from build123d import *

# Parameters (mm, degrees)
SALIENTE_EXTRUIR1_DEPTH = 10
REDONDEO1_R             = 30
REDONDEO2_R             = 150
REDONDEO3_R             = 10
CORTAR_EXTRUIR1_DEPTH   = 5
CROQUIS4_R              = 2.65
CORTAR_EXTRUIR3_DEPTH   = 5


with BuildPart() as part:
    # Croquis1 → Saliente-Extruir1 (new body)
    with BuildSketch(Plane.XY):
        Polygon((0, 0), (260, 0), (274.106158457, 80), (127.13677389, 110), (50.509014114, 286.543118386), (96.75188515, 306.61463205), (64.899290737, 380), (0, 351.830749872), align=None)
    extrude(amount=SALIENTE_EXTRUIR1_DEPTH)

    # Redondeo1
    redondeo1_edges = [part.edges().sort_by_distance(p)[0] for p in [
        (50.509014114, 286.543118386, 5),
    ]]
    fillet(redondeo1_edges, radius=REDONDEO1_R)

    # Redondeo2
    redondeo2_edges = [part.edges().sort_by_distance(p)[0] for p in [
        (127.13677389, 110, 5),
    ]]
    fillet(redondeo2_edges, radius=REDONDEO2_R)

    # Redondeo3
    redondeo3_edges = [part.edges().sort_by_distance(p)[0] for p in [
        (64.899290737, 380, 5),
        (96.75188515, 306.61463205, 5),
        (274.106158457, 80, 5),
    ]]
    fillet(redondeo3_edges, radius=REDONDEO3_R)

    # Croquis2 → Cortar-Extruir1 (cut)
    with BuildSketch(Plane.XY.offset(10)):
        Polygon((39.986675692, 287.208594669), (90.439116158, 309.107253328), (88.289066035, 314.060765665), (83.517508369, 311.989692162), (59.787325531, 366.661791285), (64.558883197, 368.732864788), (62.408833074, 373.686377124), (0, 346.598099131), (0, 340.711367047), (57.402301073, 365.626581966), (81.13248391, 310.954482844), (37.836625569, 292.162107006), align=None)
    extrude(amount=-CORTAR_EXTRUIR1_DEPTH, mode=Mode.SUBTRACT)

    # Croquis4 → Cortar-Extruir3 (cut)
    with BuildSketch(Plane.XY.offset(10)):
        with Locations((132.709363959, 88.450085292)):
            Circle(CROQUIS4_R)
        with Locations((142.50732293, 86.450085292)):
            Circle(CROQUIS4_R)
        with Locations((134.109252611, 70.308111078)):
            Circle(CROQUIS4_R)
        Polygon((254.785909436, 5), (265.569150028, 66.433298656), (260.668303978, 67.433679667), (249.709468889, 5), align=None)
        with BuildLine():
            Line((240.334745072, 17.65), (246.334745072, 17.65))
            ThreePointArc((246.334745072, 17.65), (248.984745072, 15), (246.334745072, 12.35))
            Line((246.334745072, 12.35), (240.334745072, 12.35))
            ThreePointArc((240.334745072, 12.35), (237.684745072, 15), (240.334745072, 17.65))
        make_face()
        with BuildLine():
            Line((249.552515929, 67.294739764), (255.431207696, 66.094330202))
            ThreePointArc((255.431207696, 66.094330202), (257.497449003, 62.967727115), (254.370845916, 60.901485808))
            Line((254.370845916, 60.901485808), (248.49215415, 62.10189537))
            ThreePointArc((248.49215415, 62.10189537), (246.425912843, 65.228498457), (249.552515929, 67.294739764))
        make_face()
        with BuildLine():
            Line((15, 17.65), (21, 17.65))
            ThreePointArc((21, 17.65), (23.65, 15), (21, 12.35))
            Line((21, 12.35), (15, 12.35))
            ThreePointArc((15, 12.35), (12.35, 15), (15, 17.65))
        make_face()
        Polygon((99.011814836, 96.436284415), (19.818301977, 278.890655481), (24.771814314, 281.040705604), (103.965327172, 98.586334538), align=None)
        with BuildLine():
            Line((13.6, 178.915374936), (13.6, 172.915374936))
            ThreePointArc((13.6, 172.915374936), (16.25, 170.265374936), (18.9, 172.915374936))
            Line((18.9, 172.915374936), (18.9, 178.915374936))
            ThreePointArc((18.9, 178.915374936), (16.25, 181.565374936), (13.6, 178.915374936))
        make_face()
        with BuildLine():
            Line((14.004606425, 344.282692717), (18.591191921, 346.273479867))
            ThreePointArc((18.591191921, 346.273479867), (21.879878245, 344.975580694), (20.581979072, 341.686894371))
            Line((20.581979072, 341.686894371), (15.995393575, 339.69610722))
            ThreePointArc((15.995393575, 339.69610722), (12.706707252, 340.994006393), (14.004606425, 344.282692717))
        make_face()
    extrude(amount=-CORTAR_EXTRUIR3_DEPTH, mode=Mode.SUBTRACT)


solid = part.part
Geometry: final body of the model. Coordinates: model frame, mm. A direction names the side the tool comes from. Round coordinates to 2 decimals unless told otherwise and drop trailing zeros. Order: outer loops, then holes, each group sorted by start corner. A loop starts at its lowest first (then second) coordinate and runs counter-clockwise, first axis right, second up. Notation, with made-up numbers: (-33.5, -14) -> (-28.5, -14) arc R35 ccw to (-28.5, 21) -> close; hole circle Ø2 at (5.5, 12.25). An arc over 180 degrees is marked (long way). Put each result on its own line as item: value. Start each with the question number.
Q1. Reachability of faces 5 (the flat face through (71.82, 338.94, 7.54)), 6 (the flat face through (82.737, 300.531, 4.93)), 7 (the flat face through (74, 149, 10)) from +Z, -Z, +X, -X, +Y, -Y: full face, straight path, thin tool, end or side. Return the list, or none.
Q2. Section D-D on y = 244. Return the cut outline in (x, z).
Q3. Section A-A on z = 2. Return the cut outline in (x, y).
Q4. First-contact query: pin 1 (1.6 mm diameter, centred on x = 135, y = 70.5, fed in from +Z); pin 2 (1.5 mm diameter, centred on x = 242, z = 8.5, fed in from +Y); pin 3 (6 mm diameter, centred on y = 79, z = 5.5, fed in from +X). Flat tips, straight axial feed; report the tip coordinate or a pass-through.
Q5. Section B-B on y = 202. Return the cut outline in (x, z).
Q6. Section C-C on x = 228.5. Return the cut outline in (y, z), and give its area (3 significant figures).
Q7. Line query: probe 1 along Y at (x, z) = (247, 5.75); probe 2 along X at (y, z) = (221.5, 7.25); probe 3 along X at (y, z) = (129, 1.75). Output: solid intervals per line, ascending.
Q8. Pull-direction query (X, two-part tool) for faces 1 (the flat face through (128, 0, 5)), 2 (the flat face through (31.64, 360.33, 7.54)), 3 (the flat face through (79.485, 219.784, 4.93)), 4 (the flat face through (59.79, 301.69, 7.54)); classes: +X half, -X half, draft (parallel to the pull), parting line (faces both ways), or undercut.
Ans:
1. face 5: +Z
1. face 6: +Z, -Z, +X
1. face 7: +Z, +X, -X, +Y, -Y
2. outline: (0, 0) -> (68.97, 0) -> (68.97, 10) -> (40.85, 10) -> (40.85, 5) -> (34.96, 5) -> (34.96, 10) -> (0, 10) -> close
3. outline: (0, 0) -> (260, 0) -> (272.42, 70.41) arc R10 ccw to (264.57, 81.95) -> (203.64, 94.38) arc R150 cw to (96.05, 181.63) -> (62.45, 259.02) arc R30 cw to (78.03, 298.49) -> (87.58, 302.63) arc R10 ccw to (92.77, 315.79) -> (68.88, 370.83) arc R10 ccw to (55.73, 376.02) -> (0, 351.83) -> close
4. pin 1: stops at z = 5
4. pin 2: stops at y = 86.71
4. pin 3: stops at x = 271.8
5. outline: (0, 0) -> (87.2, 0) -> (87.2, 10) -> (59.08, 10) -> (59.08, 5) -> (53.19, 5) -> (53.19, 10) -> (0, 10) -> close
6. outline: (0, 0) -> (89.31, 0) -> (89.31, 10) -> (0, 10) -> close
6. area: 893 mm2
7. probe 1: y = 0 to 12.43, 17.57 to 62.99, 66.41 to 85.53
7. probe 2: x = 0 to 44.73, 50.62 to 78.74
7. probe 3: x = 0 to 134.26
8. face 1: draft
8. face 2: undercut
8. face 3: +X half
8. face 4: undercut
